Can you work these out from the model? Positions are in its coordinate system, mm. A direction names the side the tool comes from. Give positions to 0.01 mm unless a question says otherwise; leave off trailing zeros. Loops run counter-clockwise (first coordinate to the right, second up) from the corner with the lowest first, then second, coordinate; pieces in that order, holes last. Notation, with made-up numbers: (35.25, -38) -> (84.25, -38) arc R15 ccw to (84.25, -13) -> close; hole circle Ø1 at (69.25, -7.75). An arc over 180 degrees is marked (long way). Return JSON: item names as keys, results as strings. Group by question number.
Q1. Will these pins go through, and if not, where does the flat tip stop? pin 1 (5.5 mm diameter, centred on y = 1117.6, z = -257.175, fed in from +X); pin 2 (10.5 mm diameter, centred on y = 596.9, z = -73.025, fed in from +X).
Q2. I need wall thicknesses on line 1 along Z through (x, y) = (8.5, 794); line 2 along Z through (x, y) = (9.75, 565.15); line 3 along Y through (x, z) = (6, -429.5). Which ranges of each line are inside material? Lowest first, please. Write a range as [from, to].
Q3. Suppose I cut it at C-C, the plane x = 2. Count the separate pieces of the cut face and the enclosed holes in it, and give its area (3 significant figures).
Q4. Thinking about a two-plate mould opening in Y: for faces 3 (the flat face through (0, 612, -576)), 4 (the cylindrical face through (6.261, 683.022, -309.952)), 5 (the cylindrical face through (6.261, 1082.278, -858.448)), which applies, pulls with the +Y half, pulls with the -Y half, needs draft (parallel to the pull), parting line crosses it, or undercut?
Q5. Suppose I cut it at A-A, the plane z = -589. Please give me the cut outline in (x, y).
Q6. Which directions (+Z, -Z, +X, -X, +Y, -Y) give clear straight access to the entire face, cutting with the end or side of a thin tool? Please do faces 1 (the flat face through (12.7, 612, -576)), 2 (the cylindrical face through (6.261, 684.602, -860.028)).
Q7. Suppose I cut it at B-B, the plane y = 892.5. Please give me the cut outline in (x, z), and give its area (3 significant figures).
```python
from build123d import *

# Parameters (mm, degrees)
BOSS_EXTRUDE1_DEPTH                           = 12.7
CSK_FOR_1_4_FLAT_HEAD_MACHINE_SCREW1_AT_COUNT = 2
CSK_FOR_1_4_FLAT_HEAD_MACHINE_SCREW1_AT_PITCH = 260.35
CSK_FOR_1_4_FLAT_HEAD_MACHINE_SCREW1_2_COUNT  = 2
CSK_FOR_1_4_FLAT_HEAD_MACHINE_SCREW1_2_PITCH  = 520.7
CSK_FOR_1_4_FLAT_HEAD_MACHINE_SCREW1_3_COUNT  = 2
CSK_FOR_1_4_FLAT_HEAD_MACHINE_SCREW1_3_PITCH  = 184.15
CSK_FOR_1_4_FLAT_HEAD_MACHINE_SCREW1_4_COUNT  = 2
CSK_FOR_1_4_FLAT_HEAD_MACHINE_SCREW1_4_PITCH  = 318.893940049
CSK_FOR_1_4_FLAT_HEAD_MACHINE_SCREW1_5_COUNT  = 2
CSK_FOR_1_4_FLAT_HEAD_MACHINE_SCREW1_5_PITCH  = 552.304003697
CSK_FOR_1_4_FLAT_HEAD_MACHINE_SCREW1_6_COUNT  = 2
CSK_FOR_1_4_FLAT_HEAD_MACHINE_SCREW1_6_PITCH  = 838.2
CSK_FOR_1_4_FLAT_HEAD_MACHINE_SCREW1_7_COUNT  = 2
CSK_FOR_1_4_FLAT_HEAD_MACHINE_SCREW1_7_PITCH  = 877.702319981
CSK_FOR_1_4_FLAT_HEAD_MACHINE_SCREW1_8_COUNT  = 2
CSK_FOR_1_4_FLAT_HEAD_MACHINE_SCREW1_8_PITCH  = 986.766299587
CSK_FOR_1_4_FLAT_HEAD_MACHINE_SCREW1_9_COUNT  = 2
CSK_FOR_1_4_FLAT_HEAD_MACHINE_SCREW1_9_PITCH  = 1022.35
CSK_FOR_1_4_FLAT_HEAD_MACHINE_SCREW1_10_COUNT = 2
CSK_FOR_1_4_FLAT_HEAD_MACHINE_SCREW1_10_PITCH = 1054.979452407
CSK_FOR_1_4_FLAT_HEAD_MACHINE_SCREW1_11_COUNT = 2
CSK_FOR_1_4_FLAT_HEAD_MACHINE_SCREW1_11_PITCH = 1147.313388966
F_27_64_0_42188_DIAMETER_HOLE1_D              = 10.715752


with BuildPart() as part:
    # Sketch1 → Boss-Extrude1 (new body)
    with BuildSketch(Plane(origin=(0, 0, 0), x_dir=(0, 0, -1), z_dir=(1, 0, 0))):
        with BuildLine():
            Line((6.35, 0), (1162.05, 0))
            ThreePointArc((1162.05, 0), (1166.540128061, 1.859871939), (1168.4, 6.35))
            Line((1168.4, 6.35), (1168.4, 1200.15))
            ThreePointArc((1168.4, 1200.15), (1166.540128061, 1204.640128061), (1162.05, 1206.5))
            Line((1162.05, 1206.5), (6.35, 1206.5))
            ThreePointArc((6.35, 1206.5), (1.859871939, 1204.640128061), (0, 1200.15))
            Line((0, 1200.15), (0, 6.35))
            ThreePointArc((0, 6.35), (1.859871939, 1.859871939), (6.35, 0))
        make_face()
        with BuildLine():
            Line((381, 1111.25), (787.4, 1111.25))
            ThreePointArc((787.4, 1111.25), (859.242048969, 1081.492048969), (889, 1009.65))
            Line((889, 1009.65), (889, 755.65))
            ThreePointArc((889, 755.65), (859.242048969, 683.807951031), (787.4, 654.05))
            Line((787.4, 654.05), (381, 654.05))
            ThreePointArc((381, 654.05), (309.157951031, 683.807951031), (279.4, 755.65))
            Line((279.4, 755.65), (279.4, 1009.65))
            ThreePointArc((279.4, 1009.65), (309.157951031, 1081.492048969), (381, 1111.25))
        make_face(mode=Mode.SUBTRACT)
    extrude(amount=BOSS_EXTRUDE1_DEPTH)

    # Sketch3 → CSK for 1/4 Flat Head Machine Screw1 (revolve, cut)
    with BuildSketch(Plane(origin=(12.7, 1117.6, -73.025), x_dir=(0, 0, -1), z_dir=(0, 1, 0))):
        Polygon((0, 0), (0, 12.7), (3.3782, 12.7), (3.3782, 4.536932584), (6.4389, 1.016), (6.4389, 0), align=None)
    csk_for_1_4_flat_head_machine_screw1 = revolve(axis=Axis((19.05, 1117.6, -73.025), (-1, 0, 0)), mode=Mode.SUBTRACT)

    # CSK for 1/4 Flat Head Machine Screw1 at: CSK for 1/4 Flat Head Machine Screw1 ×2
    with Locations(*[(0, -i * CSK_FOR_1_4_FLAT_HEAD_MACHINE_SCREW1_AT_PITCH, 0) for i in range(1, CSK_FOR_1_4_FLAT_HEAD_MACHINE_SCREW1_AT_COUNT)]):
        add(csk_for_1_4_flat_head_machine_screw1, mode=Mode.SUBTRACT)

    # CSK for 1_4 Flat Head Machine Screw1 2: CSK for 1/4 Flat Head Machine Screw1 ×2
    with Locations(*[(0, -i * CSK_FOR_1_4_FLAT_HEAD_MACHINE_SCREW1_2_PITCH, 0) for i in range(1, CSK_FOR_1_4_FLAT_HEAD_MACHINE_SCREW1_2_COUNT)]):
        add(csk_for_1_4_flat_head_machine_screw1, mode=Mode.SUBTRACT)

    # CSK for 1_4 Flat Head Machine Screw1 3: CSK for 1/4 Flat Head Machine Screw1 ×2
    with Locations(*[(0, 0, -i * CSK_FOR_1_4_FLAT_HEAD_MACHINE_SCREW1_3_PITCH) for i in range(1, CSK_FOR_1_4_FLAT_HEAD_MACHINE_SCREW1_3_COUNT)]):
        add(csk_for_1_4_flat_head_machine_screw1, mode=Mode.SUBTRACT)

    # CSK for 1_4 Flat Head Machine Screw1 4: CSK for 1/4 Flat Head Machine Screw1 ×2
    with Locations(*[Vector(0, -0.8164156395068651, -0.5774647206268073) * (i * CSK_FOR_1_4_FLAT_HEAD_MACHINE_SCREW1_4_PITCH) for i in range(1, CSK_FOR_1_4_FLAT_HEAD_MACHINE_SCREW1_4_COUNT)]):
        add(csk_for_1_4_flat_head_machine_screw1, mode=Mode.SUBTRACT)

    # CSK for 1_4 Flat Head Machine Screw1 5: CSK for 1/4 Flat Head Machine Screw1 ×2
    with Locations(*[Vector(0, -0.9427778841259971, -0.3334214468250479) * (i * CSK_FOR_1_4_FLAT_HEAD_MACHINE_SCREW1_5_PITCH) for i in range(1, CSK_FOR_1_4_FLAT_HEAD_MACHINE_SCREW1_5_COUNT)]):
        add(csk_for_1_4_flat_head_machine_screw1, mode=Mode.SUBTRACT)

    # CSK for 1_4 Flat Head Machine Screw1 6: CSK for 1/4 Flat Head Machine Screw1 ×2
    with Locations(*[(0, 0, -i * CSK_FOR_1_4_FLAT_HEAD_MACHINE_SCREW1_6_PITCH) for i in range(1, CSK_FOR_1_4_FLAT_HEAD_MACHINE_SCREW1_6_COUNT)]):
        add(csk_for_1_4_flat_head_machine_screw1, mode=Mode.SUBTRACT)

    # CSK for 1_4 Flat Head Machine Screw1 7: CSK for 1/4 Flat Head Machine Screw1 ×2
    with Locations(*[Vector(0, -0.2966267652176661, -0.9549934880178522) * (i * CSK_FOR_1_4_FLAT_HEAD_MACHINE_SCREW1_7_PITCH) for i in range(1, CSK_FOR_1_4_FLAT_HEAD_MACHINE_SCREW1_7_COUNT)]):
        add(csk_for_1_4_flat_head_machine_screw1, mode=Mode.SUBTRACT)

    # CSK for 1_4 Flat Head Machine Screw1 8: CSK for 1/4 Flat Head Machine Screw1 ×2
    with Locations(*[Vector(0, -0.5276832014004726, -0.8494412510349073) * (i * CSK_FOR_1_4_FLAT_HEAD_MACHINE_SCREW1_8_PITCH) for i in range(1, CSK_FOR_1_4_FLAT_HEAD_MACHINE_SCREW1_8_COUNT)]):
        add(csk_for_1_4_flat_head_machine_screw1, mode=Mode.SUBTRACT)

    # CSK for 1_4 Flat Head Machine Screw1 9: CSK for 1/4 Flat Head Machine Screw1 ×2
    with Locations(*[(0, 0, -i * CSK_FOR_1_4_FLAT_HEAD_MACHINE_SCREW1_9_PITCH) for i in range(1, CSK_FOR_1_4_FLAT_HEAD_MACHINE_SCREW1_9_COUNT)]):
        add(csk_for_1_4_flat_head_machine_screw1, mode=Mode.SUBTRACT)

    # CSK for 1_4 Flat Head Machine Screw1 10: CSK for 1/4 Flat Head Machine Screw1 ×2
    with Locations(*[Vector(0, -0.2467820576089035, -0.9690710067081337) * (i * CSK_FOR_1_4_FLAT_HEAD_MACHINE_SCREW1_10_PITCH) for i in range(1, CSK_FOR_1_4_FLAT_HEAD_MACHINE_SCREW1_10_COUNT)]):
        add(csk_for_1_4_flat_head_machine_screw1, mode=Mode.SUBTRACT)

    # CSK for 1_4 Flat Head Machine Screw1 11: CSK for 1/4 Flat Head Machine Screw1 ×2
    with Locations(*[Vector(0, -0.4538428689212819, -0.891081730443005) * (i * CSK_FOR_1_4_FLAT_HEAD_MACHINE_SCREW1_11_PITCH) for i in range(1, CSK_FOR_1_4_FLAT_HEAD_MACHINE_SCREW1_11_COUNT)]):
        add(csk_for_1_4_flat_head_machine_screw1, mode=Mode.SUBTRACT)

    # 27/64 (0.42188) Diameter Hole1 (through all)
    with Locations(Plane(origin=(12.7, 0, 0), x_dir=(0, 0, -1), z_dir=(1, 0, 0))):
        with Locations((22.225, 1047.75), (22.225, 1022.35), (22.225, 819.15), (22.225, 793.75), (22.225, 590.55), (22.225, 565.15), (1146.175, 1047.75), (1146.175, 1022.35), (1146.175, 819.15), (1146.175, 793.75), (1146.175, 565.15), (1146.175, 590.55)):
            Hole(F_27_64_0_42188_DIAMETER_HOLE1_D / 2)


solid = part.part
```
Ans:
{
 "1": {"pin 1": "passes through", "pin 2": "stops at x = 10.32"},
 "2": {"line 1": "z = [-1168.4, -1151.53], [-1140.82, -889], [-279.4, -27.58], [-16.87, 0]", "line 2": "z = [-1168.4, -1151.53], [-1140.82, -27.58], [-16.87, 0]", "line 3": "y = [0, 654.05], [1111.25, 1206.5]"},
 "3": {"separate pieces": "1", "enclosed holes": "25", "area": "1,140,000 mm^2"},
 "4": {"face 3": "needs draft", "face 4": "undercut", "face 5": "undercut"},
 "5": {"outline": "(0, 0) -> (12.7, 0) -> (12.7, 654.05) -> (0, 654.05) -> close; (0, 1111.25) -> (12.7, 1111.25) -> (12.7, 1206.5) -> (0, 1206.5) -> close"},
 "6": {"face 1": "+Z, -Z, +X, +Y, -Y", "face 2": "+X, -X"},
 "7": {"outline": "(0, -1168.4) -> (12.7, -1168.4) -> (12.7, -889) -> (0, -889) -> close; (0, -279.4) -> (12.7, -279.4) -> (12.7, 0) -> (0, 0) -> close", "area": "7,100 mm^2"}
}
